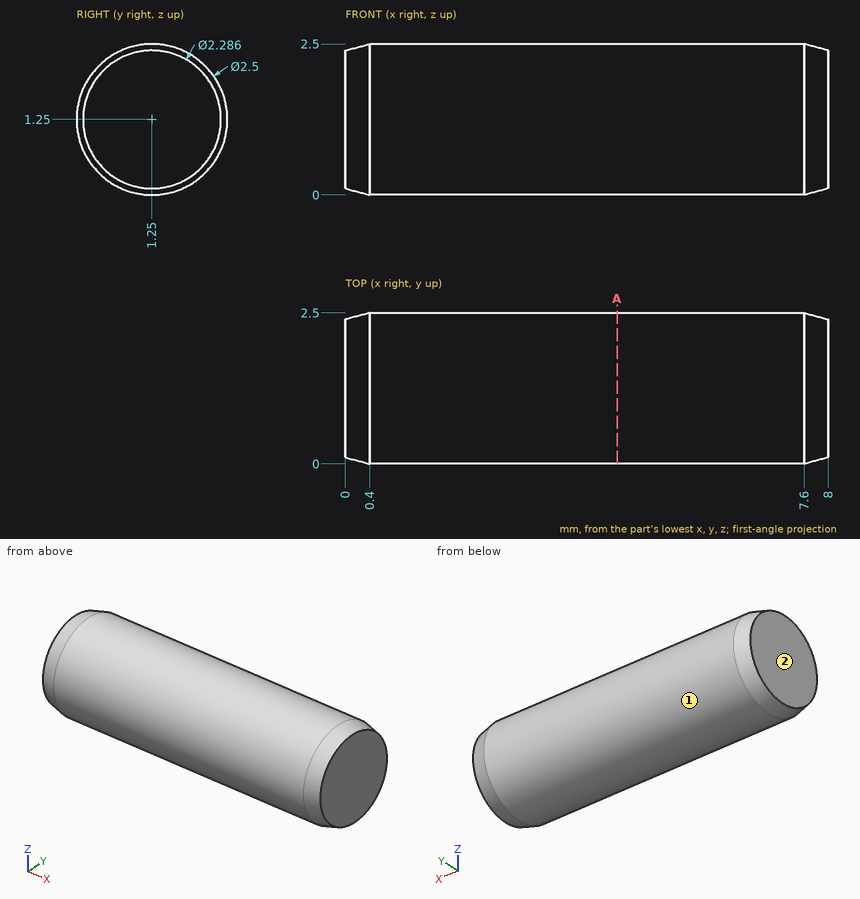
Verification items for this drawing (mm, ordinates from the low corner). Coordinates: 2 decimals unless noted, no trailing zeros. Loops run counter-clockwise (first coordinate to the right, second up) from the corner with the lowest first, then second, coordinate; pieces in that order, holes last. Notation, with made-up numbers: (-24, 40.5) - (11, 40.5) arc R8 ccw to (11, 48.5) - close; hole circle Ø3 at (-23.5, 32.5). An arc over 180 degrees is marked (long way). One line per item, written item: value. Start each with the question number.
(1) Material ranges on line 1 (Y direction, x = 3, z = 1.3); line 2 (Z direction, x = 1, y = 0.6), recorded low to high. Write a range as [from, to].
(2) Cross-section at A-A on x = 4.5. Enter the section's corners in (y, z).
(3) Mould release check, pull along Z, two halves, no side actions. Record for the marked faces 1 and 2: released by +Z, released by -Z, zero draft, split by the parting line, or undercut.
Results below:
1. line 1: y = [0, 2.5]
1. line 2: z = [0.18, 2.32]
2. outline: circle Ø2.5 at (1.25, 1.25)
3. face 1: split by the parting line
3. face 2: zero draft
